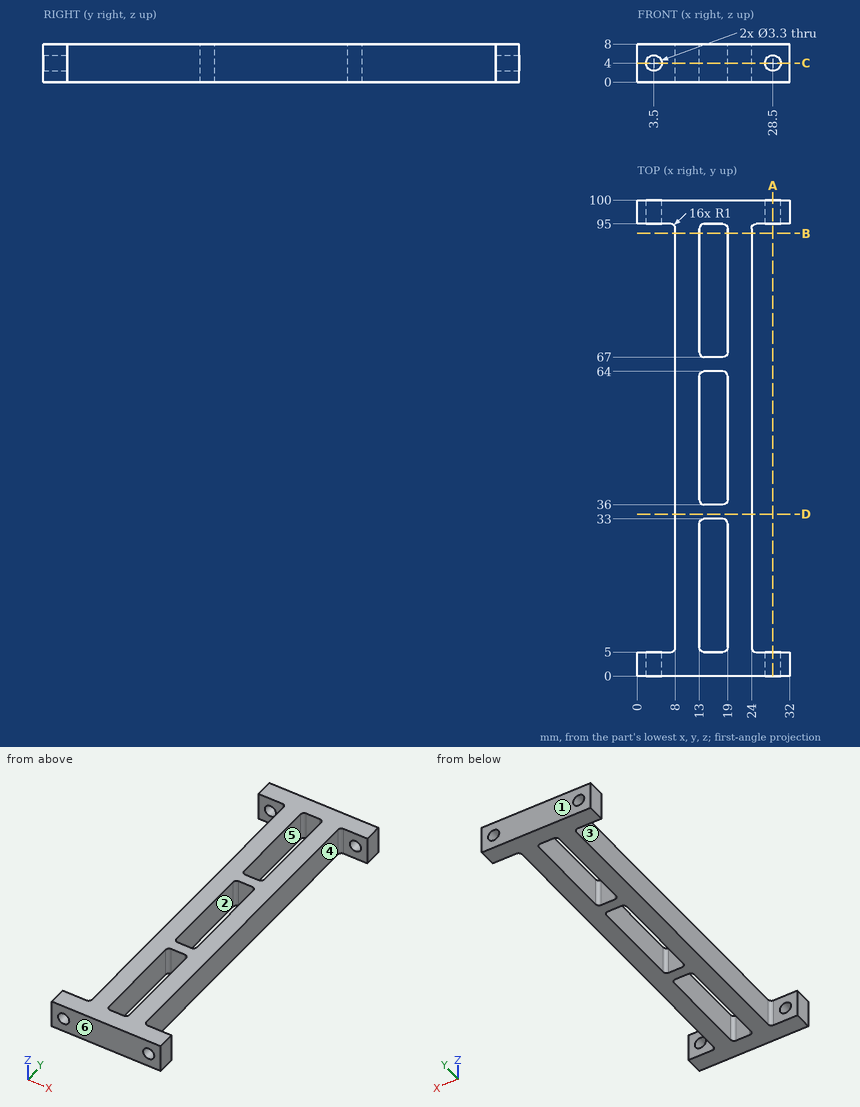
Print and shaded views of the part. All mm, measured from the part's lowest x, y and z. A direction names the side the tool comes from. Coordinates: 2 decimals unless noted, no trailing zeros. Order: outer loops, then holes, each group sorted by start corner. A loop starts at its lowest first (then second) coordinate and runs counter-clockwise, first axis right, second up. Notation, with made-up numbers: M 60.5,10 L 97.5,10 A24 ccw 97.5,36 Z; hole C -7.75,60 d11. An arc over 180 degrees is marked long. One line per question, with ' | ' between items. Start each with the question number.
Q1. Saw through at A-A (x = 28.5). List the corners of the cut face in (y, z).
Q2. Probe L1, parallel to X at y = 3.15, z = 4; L2, parallel to Y at x = 15.5, z = 4.25; L3, parallel to X at y = 85.5, z = 5. List the from-to ranges inside material, lowest first. Write a range as from..to.
Q3. Saw through at C-C (z = 4). Count the separate pieces of the cut face and the enclosed holes in it, then the cut area to 3 significant figures.
Q4. 3-axis set-ups, long thin cutter, end or side, ignore diameter. For the marked faces 1, 2 and 3: which of +Z, -Z, +X, -X, +Y, -Y reach the whole face in a straight line?
Q5. Flat gauge pins, fed straight in: pin 1 Ø3.5 at (x, z) = (30, 4.5) entering from -Y; pin 2 Ø1 at (y, z) = (74.5, 4) entering from -X; pin 3 Ø2.5 at (x, z) = (3.5, 4) entering from +Y; pin 4 Ø4 at (y, z) = (21.5, 2) entering from +X. Where does each tip first touch, or does it go through?
Q6. Two-plate mould, pull along X, no slides. Class the marked faces 4, 5 and 6: +X half, -X half, draft (parallel to the pull), parting line (faces both ways), or undercut.
Q7. Saw through at B-B (y = 93). List the corners of the cut face in (x, z).
Q8. Saw through at D-D (y = 34). List the corners of the cut face in (x, z).
Check values:
1) outline: M 0,0 L 5,0 L 5,2.35 L 0,2.35 Z; M 0,5.65 L 5,5.65 L 5,8 L 0,8 Z; M 95,0 L 100,0 L 100,2.35 L 95,2.35 Z; M 95,5.65 L 100,5.65 L 100,8 L 95,8 Z
2) L1: x = 0..1.85, 5.15..26.85, 30.15..32 | L2: y = 0..5, 33..36, 64..67, 95..100 | L3: x = 8..13, 19..24
3) separate pieces: 5 | enclosed holes: 3 | area: 1,190 mm2
4) face 1: +Z, -Z, +X, -X, +Y | face 2: +Z, -Z | face 3: +Z, -Z, -X
5) pin 1: stops at y = 0 | pin 2: stops at x = 8 | pin 3: passes through | pin 4: stops at x = 24
6) face 4: +X half | face 5: undercut | face 6: draft
7) outline: M 8,0 L 13,0 L 13,8 L 8,8 Z; M 19,0 L 24,0 L 24,8 L 19,8 Z
8) outline: M 8,0 L 24,0 L 24,8 L 8,8 Z
